from build123d import *

# Parameters (mm, degrees)
SKETCH2_R           = 1
BODY_DEPTH          = 2.9
LEVER_DEPTH         = 1.8
LEGS_DEPTH          = 0.27
BOSS_EXTRUDE3_DEPTH = 1.375


# Sheet-metal steps are written as plain solids
with BuildPart() as part:
    # Sketch2 → Body (new, symmetric)
    with BuildSketch(Plane.XY):
        Polygon((-6.3, -3.05), (-4.65, -3.05), (-4.65, -3.55), (-2.25, -3.55), (-2.25, -3.05), (2.25, -3.05), (2.25, -3.55), (4.65, -3.55), (4.65, -3.05), (6.3, -3.05), (6.3, 3.05), (-6.3, 3.05), align=None)
        with Locations((-3.45, -2.05)):
            Circle(SKETCH2_R, mode=Mode.SUBTRACT)
        with Locations((3.45, -2.05)):
            Circle(SKETCH2_R, mode=Mode.SUBTRACT)
    extrude(amount=BODY_DEPTH, both=True)

    # Sketch8 → Legs (add, symmetric)
    with BuildSketch(Plane.XY):
        Polygon((-4.705, -3.05), (-5.455, -3.05), (-5.455, -5.94846389), (-5.126348987, -6.45), (-5.033651013, -6.45), (-4.705, -5.94846389), align=None)
        Polygon((0.375, -3.05), (-0.375, -3.05), (-0.375, -5.94846389), (-0.046348987, -6.45), (0.046348987, -6.45), (0.375, -5.94846389), align=None)
        Polygon((5.455, -3.05), (4.705, -3.05), (4.705, -5.94846389), (5.033651013, -6.45), (5.126348987, -6.45), (5.455, -5.94846389), align=None)
    extrude(amount=LEGS_DEPTH, both=True)



with BuildPart() as body_2:
    # Sketch3 → Lever (new, symmetric)
    with BuildSketch(Plane.XY):
        with BuildLine():
            Line((-5.3, 3.05), (-5.3, 3.210873935))
            ThreePointArc((-5.3, 3.210873935), (-5.206775112, 3.474726216), (-4.96848559, 3.621447071))
            Line((-4.96848559, 3.621447071), (7.603727147, 6.330975678))
            Line((7.603727147, 6.330975678), (7.671144739, 6.01815805))
            Line((7.671144739, 6.01815805), (-4.901067998, 3.308629443))
            ThreePointArc((-4.901067998, 3.308629443), (-4.957803598, 3.273695906), (-4.98, 3.210873935))
            Line((-4.98, 3.210873935), (-4.98, 3.05))
            Line((-4.98, 3.05), (-5.3, 3.05))
        make_face()
    extrude(amount=LEVER_DEPTH, both=True)


with BuildPart() as part_1:
    add(part.part)

    add(body_2.part)  # Boss-Extrude3 merges body 2
    # Sketch9 → Boss-Extrude3 (add, symmetric)
    with BuildSketch(Plane.XY):
        with BuildLine():
            Line((-2.6, 3.05), (-2.6, 3.55))
            ThreePointArc((-2.6, 3.55), (-2.1, 4.05), (-1.6, 3.55))
            Line((-1.6, 3.55), (-1.6, 3.05))
            Line((-1.6, 3.05), (-2.6, 3.05))
        make_face()
    extrude(amount=BOSS_EXTRUDE3_DEPTH, both=True)


solid = part_1.part
Here's how the part is built. I have some questions about the finished solid (model axes, mm). A direction names the side the tool comes from. Give positions to 0.01 mm unless a question says otherwise; leave off trailing zeros. Loops run counter-clockwise (first coordinate to the right, second up) from the corner with the lowest first, then second, coordinate; pieces in that order, holes last. Notation, with made-up numbers: (-10, 30) -> (6, 30) arc R18 cw to (6, 48) -> close; hole circle Ø11 at (20, -17.75). An arc over 180 degrees is marked (long way). Answer as a JSON object with one key per item and string values. Group by question number.
Item 1: Imagine slicing it at C-C on z = -2.4. Write out the boundary of the cut face in (x, y).
Item 2: On a 3-axis mill with a long thin cutter (end or side, diameter ignored), from which of +Z, -Z, +X, -X, +Y, -Y can I reach the whole of each face in a straight line? I mean faces 1 (the flat face through (1.7, 4.9, -1.8)), 2 (the flat face through (-2.1, 3.5, -1.375)), 3 (the flat face through (-2.1, 3.5, 1.375)), 4 (the flat face through (6.3, 0, 0)). Say none if no direction works.
Item 3: Imagine slicing it at D-D on x = 5.75. Write out the boundary of the cut face in (y, z).
Item 4: I need wall thicknesses on L1, parallel to Y at x = 3.5, z = -1.3; L2, parallel to X at y = 2.75, z = -2.4; L3, parallel to Y at x = -3.45, z = 1.75. Which ranges of each line are inside material? Lowest first, please.
Item 5: Imagine slicing it at A-A on z = -0.9. Write out the boundary of the cut face in (x, y), then the cut area to 3 significant figures.
Item 6: Thinking about a two-plate mould opening in Y: for faces 5 (the flat face through (-3, -3.55, 0)), 6 (the flat face through (0, 3.05, 0)), 7 (the flat face through (1.7, 4.9, 1.8)), which applies, pulls with the +Y half, pulls with the -Y half, needs draft (parallel to the pull), parting line crosses it, or undercut?
Item 7: Imagine slicing it at B-B on y = -2.05. Write out the boundary of the cut face in (x, z).
Item 8: Will these pins go through, and if not, where does the flat tip stop? pin 1 (0.7 mm diameter, centred on x = 3, z = 0.5, fed in from -Y); pin 2 (3 mm diameter, centred on y = 0.5, z = 0, fed in from +X); pin 3 (0.6 mm diameter, centred on y = -4.5, z = 0, fed in from -X) (3 decimals).
Answer list:
{
 "1": {"outline": "(-6.3, -3.05) -> (-4.65, -3.05) -> (-4.65, -3.55) -> (-2.25, -3.55) -> (-2.25, -3.05) -> (2.25, -3.05) -> (2.25, -3.55) -> (4.65, -3.55) -> (4.65, -3.05) -> (6.3, -3.05) -> (6.3, 3.05) -> (-6.3, 3.05) -> close; hole circle Ø2 at (-3.45, -2.05); hole circle Ø2 at (3.45, -2.05)"},
 "2": {"face 1": "-Z, +X, -X, +Y", "face 2": "-Z, +X", "face 3": "+Z, +X", "face 4": "+Z, -Z, +X, -Y"},
 "3": {"outline": "(-3.05, -2.9) -> (3.05, -2.9) -> (3.05, 2.9) -> (-3.05, 2.9) -> close; (5.6, -1.8) -> (5.93, -1.8) -> (5.93, 1.8) -> (5.6, 1.8) -> close"},
 "4": {"L1": "y = -3.55 to -3.05, -1.05 to 3.05, 5.12 to 5.45", "L2": "x = -6.3 to 6.3", "L3": "y = -3.55 to -3.05, -1.05 to 3.05, 3.62 to 3.95"},
 "5": {"outline": "(-6.3, -3.05) -> (-4.65, -3.05) -> (-4.65, -3.55) -> (-2.25, -3.55) -> (-2.25, -3.05) -> (2.25, -3.05) -> (2.25, -3.55) -> (4.65, -3.55) -> (4.65, -3.05) -> (6.3, -3.05) -> (6.3, 3.05) -> (-1.6, 3.05) -> (-1.6, 3.55) arc R0.5 ccw to (-1.83, 3.97) -> (7.67, 6.02) -> (7.6, 6.33) -> (-4.97, 3.62) arc R0.42 ccw to (-5.3, 3.21) -> (-5.3, 3.05) -> (-6.3, 3.05) -> close; hole (-4.98, 3.05) -> (-2.6, 3.05) -> (-2.6, 3.55) arc R0.5 cw to (-2.52, 3.82) -> (-4.9, 3.31) arc R0.1 ccw to (-4.98, 3.21) -> close; hole circle Ø2 at (-3.45, -2.05); hole circle Ø2 at (3.45, -2.05)", "area": "78.1 mm2"},
 "6": {"face 5": "pulls with the -Y half", "face 6": "undercut", "face 7": "needs draft"},
 "7": {"outline": "(-6.3, -2.9) -> (-4.45, -2.9) -> (-4.45, 2.9) -> (-6.3, 2.9) -> close; (-2.45, -2.9) -> (2.45, -2.9) -> (2.45, 2.9) -> (-2.45, 2.9) -> close; (4.45, -2.9) -> (6.3, -2.9) -> (6.3, 2.9) -> (4.45, 2.9) -> close"},
 "8": {"pin 1": "stops at y = -3.55", "pin 2": "stops at x = 6.3", "pin 3": "stops at x = -5.455"}
}
